Part print with two shaded views. Sizes in mm from the minimum x, y, z corner. Coordinates: 2 decimals unless noted, no trailing zeros. Loops run counter-clockwise (first coordinate to the right, second up) from the corner with the lowest first, then second, coordinate; pieces in that order, holes last. Notation, with made-up numbers: (15.25, 25.25) -> (56.25, 25.25) arc R14 cw to (56.25, 43.25) -> close; hole circle Ø11 at (75.5, 77.25). An arc over 180 degrees is marked (long way). Return JSON: item names as keys, results as strings. Group by question number.
(1) Saw through at C-C on z = 70. Write the cut outline in (x, y).
(2) Flat gauge pin, fed straight in: pin 1 Ø10 at (x, z) = (227.5, 92) entering from +Y. Where does the tip first touch, or does it go through?
(3) Probe L1, parallel to X at y = 1.25, z = 79; L2, parallel to Z at x = 133, y = 2.5; L3, parallel to Z at x = 191.5, y = 7.5. List the from-to ranges inside material, lowest first.
(4) Saw through at B-B on x = 180. Write the cut outline in (y, z), then the cut area to 4 significant figures.
(5) Mould opens along X. For the marked faces 1 and 2 say: pulls with the +X half, pulls with the -X half, needs draft (parallel to the pull), parting line crosses it, or undercut.
(6) Saw through at A-A on y = 3.5. Write the cut outline in (x, z).
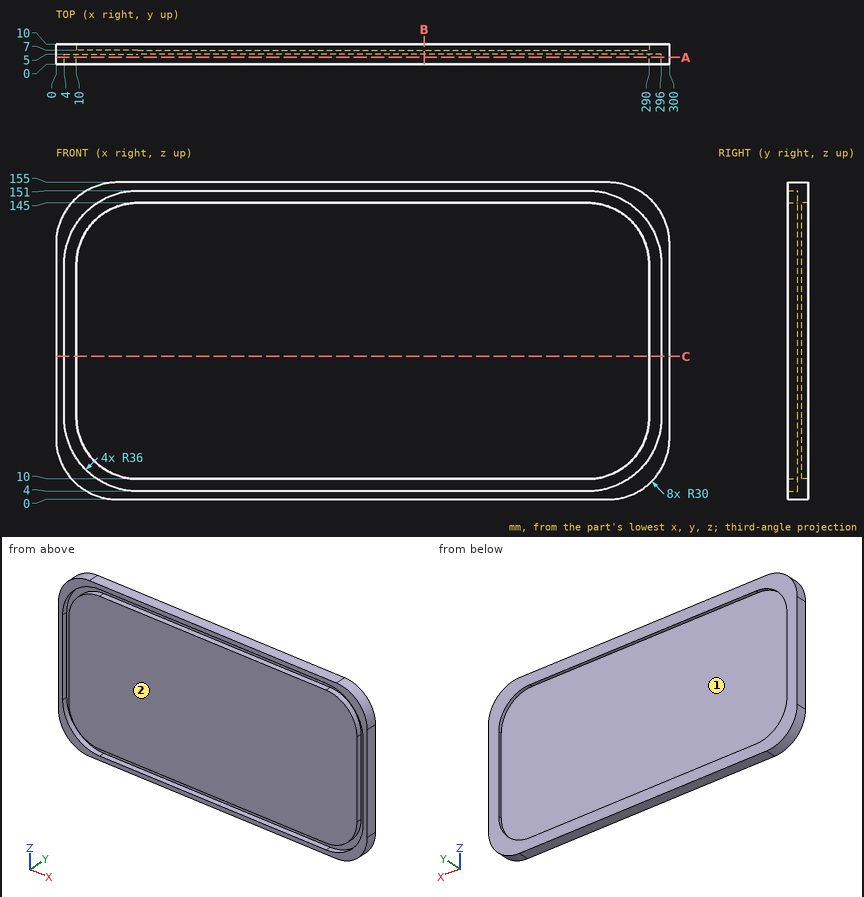
Geometry results:
{
 "1": {"outline": "(0, 0) -> (4, 0) -> (4, 5) -> (10, 5) -> (10, 0) -> (290, 0) -> (290, 5) -> (296, 5) -> (296, 0) -> (300, 0) -> (300, 10) -> (290, 10) -> (290, 7) -> (10, 7) -> (10, 10) -> (0, 10) -> close"},
 "2": {"pin 1": "y = 7"},
 "3": {"L1": "0 to 4, 10 to 290, 296 to 300", "L2": "0 to 4, 10 to 145, 151 to 155", "L3": "0 to 10, 145 to 155"},
 "4": {"outline": "(0, 0) -> (10, 0) -> (10, 10) -> (7, 10) -> (7, 145) -> (10, 145) -> (10, 155) -> (0, 155) -> (0, 151) -> (5, 151) -> (5, 145) -> (0, 145) -> (0, 10) -> (5, 10) -> (5, 4) -> (0, 4) -> close", "area": "1,085 mm²"},
 "5": {"face 1": "undercut", "face 2": "needs draft"},
 "6": {"outline": "(0, 30) arc R30 ccw to (30, 0) -> (270, 0) arc R30 ccw to (300, 30) -> (300, 125) arc R30 ccw to (270, 155) -> (30, 155) arc R30 ccw to (0, 125) -> close; (10, 40) arc R30 ccw to (40, 10) -> (260, 10) arc R30 ccw to (290, 40) -> (290, 115) arc R30 ccw to (260, 145) -> (40, 145) arc R30 ccw to (10, 115) -> close; hole (4, 40) arc R36 ccw to (40, 4) -> (260, 4) arc R36 ccw to (296, 40) -> (296, 115) arc R36 ccw to (260, 151) -> (40, 151) arc R36 ccw to (4, 115) -> close"}
}
